The model under review builds one solid part; all positions refer to its coordinate system, in mm. A direction names the side the tool comes from. Coordinates: 2 decimals unless noted, no trailing zeros. Order: outer loops, then holes, each group sorted by start corner. A loop starts at its lowest first (then second) coordinate and runs counter-clockwise, first axis right, second up. Notation, with made-up numbers: M 48,65.5 L 83,65.5 A29 ccw 83,103.5 Z; hole C -7,25 d2. An arc over 180 degrees is marked long. One line per item, written item: value.
```python
from build123d import *


# Read off the part's stored shape, not the designer's step: 3/8-16 机械螺纹 螺柱1
with BuildPart() as part:
    # 草图1 → 旋转3 (revolve)
    with BuildSketch(Plane.XY, mode=Mode.PRIVATE) as revolve_3_sk:
        Polygon((0, 0), (0, 14), (-4, 14), (-5, 12), (-5, 0), align=None)
    revolve(revolve_3_sk.sketch.rotate(Axis((0, 0, 0), (0, 1, 0)), 270), axis=Axis((0, 0, 0), (0, 1, 0)))

    # 3/8-16 机械螺纹 螺柱1 outline → 3/8-16 机械螺纹 螺柱1 (revolve, cut)
    with BuildSketch(Plane.XY):
        Polygon((3.81635, 0), (5, 0), (5, 10), (4.7625, 10), (4.7625, 0.94615), align=None)
    revolve(axis=Axis((0, 0, 0), (0, 1, 0)), mode=Mode.SUBTRACT)


solid = part.part
```
(1) We need section A-A, the plane z = 0. State the section outline as (x, y) points, plus the area to 3 significant figures.
Geometry results:
outline: M -5,10 L -4.76,10 L -4.76,0.95 L -3.82,0 L 3.82,0 L 4.76,0.95 L 4.76,10 L 5,10 L 5,12 L 4,14 L -4,14 L -5,12 Z
area: 132 mm2
(2) Insertion check: pin 1 Ø1.5 at (x, z) = (-2, -1.5) entering from -Y; pin 2 Ø6 at (y, z) = (5.5, -1.5) entering from +X; pin 3 Ø1.5 at (x, y) = (2, 2.5) entering from +Z. Each pin has a flat end and moves straight along its axis. Give the tip position at first contact, or say it passes through.
Geometry results:
pin 1: stops at y = 0
pin 2: stops at x = 4.76
pin 3: stops at z = 4.6
(3) We need section D-D, the plane y = 10.75. State the section outline as (x, z) points.
Geometry results:
outline: C 0,0 d10
(4) For L1, parallel to Z at x = 1, y = 11.5; L2, parallel to Z at x = 0.25, y = 8.5; L3, parallel to X at y = 7, z = 4.25, list the stretches that pass through material, from the lowest coordinate up.
Geometry results:
L1: z = -4.9 to 4.9
L2: z = -4.76 to 4.76
L3: x = -2.15 to 2.15
(5) We need section C-C, the plane y = 7.5. State the section outline as (x, z) points (1 decimal), plus the area to 3 significant figures.
Geometry results:
outline: C 0,0 d9.5
area: 71.3 mm2
(6) Tool access review of faces 1 (the cylindrical face through (-3.78, 5.41, 2.9)), 2 (the flat face through (0, 14, 0)): name each direction out of +Z, -Z, +X, -X, +Y, -Y from which nothing blocks a thin tool from reaching the whole face with its end or side.
Geometry results:
face 1: -Y
face 2: +Z, -Z, +X, -X, +Y
(7) We need section B-B, the plane x = 0. State the section outline as (y, z) points.
Geometry results:
outline: M 0,-3.82 L 0.95,-4.76 L 10,-4.76 L 10,-5 L 12,-5 L 14,-4 L 14,4 L 12,5 L 10,5 L 10,4.76 L 0.95,4.76 L 0,3.82 Z
